Read the model definition and answer for the solid it produces. Units are mm, in the model's axes. A direction names the side the tool comes from. Give positions to 0.01 mm unless a question says otherwise; leave off trailing zeros. Write each loop counter-clockwise with the first axis right and the second up, starting at its lowest first coordinate (ties: lowest second). Pieces come first, ordered by that corner, then holes. Notation, with made-up numbers: (84, -34.5) -> (100, -34.5) arc R29 ccw to (100, -5.5) -> close; hole circle Ø11 at (-25, 79.5). An arc over 180 degrees is marked (long way). Put each result on its own line as item: value. Start each with the question number.
from build123d import *

# Parameters (mm, degrees)
F0_W     = 450
F0_H     = 350
F1_DEPTH = 450
F2_T     = -25
F3_R     = 4
F4_DEPTH = 450.001


with BuildPart() as f1:
    # F0 (on Front) → F1 (new body)
    with BuildSketch(Plane.XZ):
        Rectangle(F0_W, F0_H)
    extrude(amount=F1_DEPTH)

    # F2
    f2_openings = [f1.faces().sort_by_distance(p)[0] for p in [
        (0, -450, 0),
    ]]
    offset(amount=F2_T, openings=f2_openings)

    # F3 (on face) → F4 (cut, through all)
    with BuildSketch(Plane(origin=(0, 0, 0), x_dir=(-1, 0, 0), z_dir=(0, 1, 0))):
        Circle(F3_R)
    extrude(amount=-F4_DEPTH, mode=Mode.SUBTRACT)


solid = f1.part
1) For a pull along Z with two mould halves and no side action, classify faces 1 (the face through (-3, -222, -175)), 2 (the face through (-200, -235, -2)), 3 (the face through (-3, -222, 175)) as pulls with the +Z half, pulls with the -Z half, needs draft (parallel to the pull), parting line crosses it, or undercut.
2) Straight lines are drawn through the part: line 1 (X direction, y = -407, z = 105); line 2 (Z direction, x = 0, y = -10.5); line 3 (Z direction, x = -117.5, y = -218.5). For each, find the intervals that lie inside material, in ascending order. Write a range as [from, to].
3) A cutting plane is placed at A-A on y = -228. Give the vertices of the cut face in (x, z), and give its area (3 significant figures).
4) For faces 4 (the face through (-3, -235, 150)), 5 (the face through (-51, -450, -155)), determine the directions among +Z, -Z, +X, -X, +Y, -Y from which every point of the face is accessible in a straight line to the end or side of a thin tool.
5) A cutting plane is placed at C-C on x = 75.5. Give the vertices of the cut face in (y, z), and give its area (3 significant figures).
6) A cutting plane is placed at B-B on z = 127.5. Give the vertices of the cut face in (x, y).
7) This flat-tipped pin is pushed along its axis until it touches: pin 1 Ø6 at (x, z) = (-177, 87.5) entering from -Y. Where does it stop, or does it pass through?
Results found:
1. face 1: pulls with the -Z half
1. face 2: undercut
1. face 3: pulls with the +Z half
2. line 1: x = [-225, -200], [200, 225]
2. line 2: z = [-175, -4], [4, 175]
2. line 3: z = [-175, -150], [150, 175]
3. outline: (-225, -175) -> (225, -175) -> (225, 175) -> (-225, 175) -> close; hole (-200, -150) -> (200, -150) -> (200, 150) -> (-200, 150) -> close
3. area: 37,500 mm²
4. face 4: -Y
4. face 5: +Z, -Z, +X, -X, -Y
5. outline: (-450, -175) -> (0, -175) -> (0, 175) -> (-450, 175) -> (-450, 150) -> (-25, 150) -> (-25, -150) -> (-450, -150) -> close
5. area: 30,000 mm²
6. outline: (-225, -450) -> (-200, -450) -> (-200, -25) -> (200, -25) -> (200, -450) -> (225, -450) -> (225, 0) -> (-225, 0) -> close
7. pin 1: stops at y = -25
